Drawing for the job (mm, zero at the part's lowest x, y, z). Coordinates: 2 decimals unless noted, no trailing zeros. Loops run counter-clockwise (first coordinate to the right, second up) from the corner with the lowest first, then second, coordinate; pieces in that order, holes last. Notation, with made-up numbers: (17.25, 41) - (56.25, 41) arc R4 cw to (56.25, 48) - close; hole circle Ø11 at (73, 29.25). An arc over 180 degrees is marked (long way). One line per item, written item: value.
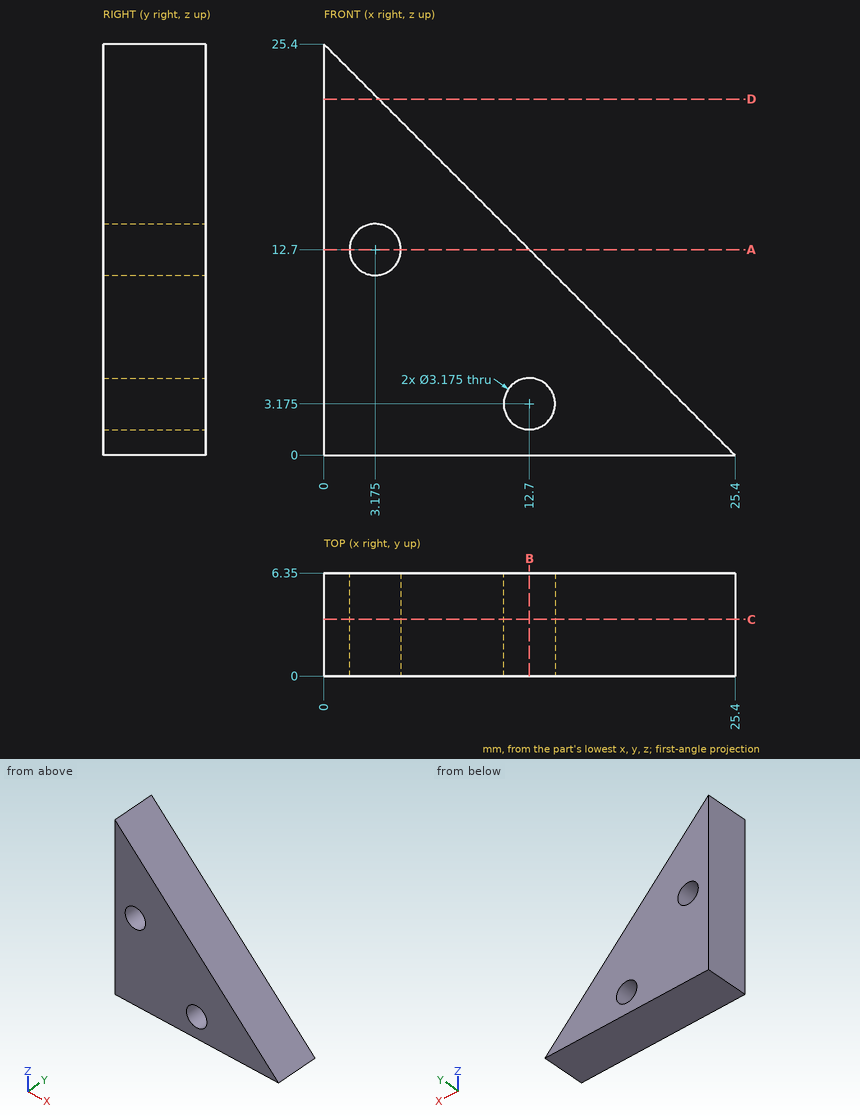
Item 1: Drop flat-ended pins along their axis: P1, Ø1.5, axis at x = 6, y = 1, coming from the +Z side; P2, Ø1.9, axis at x = 12.7, z = 3.175, coming from the -Y side; P3, Ø3, axis at y = 5.5, z = 8, coming from the +X side. Give the stop position or say it passes through.
Check result:
P1: stops at z = 20.15
P2: passes through
P3: stops at x = 18.9
Item 2: Cut at A-A, the plane z = 12.7. Write the cut outline in (x, y).
Check result:
outline: (0, 0) - (1.59, 0) - (1.59, 6.35) - (0, 6.35) - close; (4.76, 0) - (12.7, 0) - (12.7, 6.35) - (4.76, 6.35) - close
Item 3: Cut at D-D, the plane z = 22. Write the cut outline in (x, y).
Check result:
outline: (0, 0) - (3.4, 0) - (3.4, 6.35) - (0, 6.35) - close
Item 4: Probe probe 1 along Z at (x, y) = (4, 5); probe 2 along Z at (x, y) = (11.25, 1.5); probe 3 along X at (y, z) = (5.75, 8.75). List the from-to ranges inside material, lowest first. Write a range as from..to.
Check result:
probe 1: z = 0..11.34, 14.06..21.4
probe 2: z = 0..2.53, 3.82..14.15
probe 3: x = 0..16.65
Item 5: Cut at B-B, the plane x = 12.7. Write the cut outline in (y, z).
Check result:
outline: (0, 0) - (6.35, 0) - (6.35, 1.59) - (0, 1.59) - close; (0, 4.76) - (6.35, 4.76) - (6.35, 12.7) - (0, 12.7) - close
Item 6: Cut at C-C, the plane y = 3.5. Write the cut outline in (x, z) (1 decimal).
Check result:
outline: (0, 0) - (25.4, 0) - (0, 25.4) - close; hole circle Ø3.2 at (3.2, 12.7); hole circle Ø3.2 at (12.7, 3.2)
